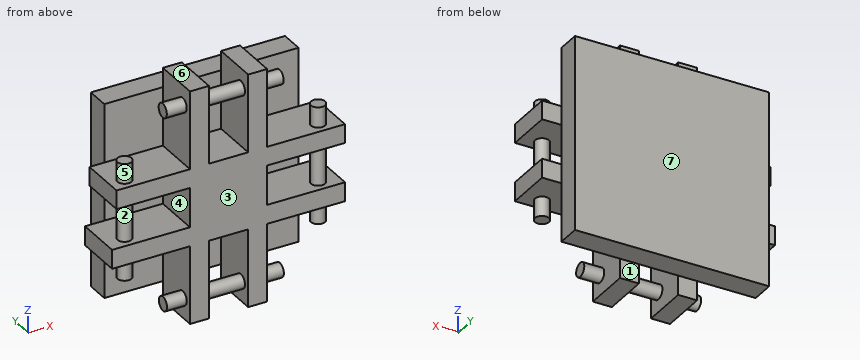
from build123d import *

# Parameters (mm, degrees)
SKETCH1_W                = 79.8
SKETCH1_H                = 79.8
BOSS_EXTRUDE1_DEPTH      = 9.6
SKETCH3_W                = 93.857769302
SKETCH3_H                = 7.7
SKETCH3_W_2              = 31.7
SKETCH3_H_2              = 31.7
SKETCH3_W_3              = 95.7
SKETCH3_H_3              = 7.8
SKETCH3_W_4              = 7.8
SKETCH3_H_4              = 95.7
BOSS_EXTRUDE2_DEPTH      = 19.3
BOSS_EXTRUDE3_DEPTH      = 32
BOSS_EXTRUDE3_DEPTH_BACK = 16
SKETCH4_R                = 2.9
BOSS_EXTRUDE4_DEPTH      = 32
BOSS_EXTRUDE4_DEPTH_BACK = 16
SKETCH5_R                = 2.9
BOSS_EXTRUDE5_DEPTH      = 32
BOSS_EXTRUDE5_DEPTH_BACK = 16
SKETCH6_R                = 2.9
BOSS_EXTRUDE6_DEPTH      = 32
BOSS_EXTRUDE6_DEPTH_BACK = 16
SKETCH7_R                = 2.9


with BuildPart() as part:
    # Sketch1 → Boss-Extrude1 (new body)
    with BuildSketch(Plane(origin=(0, 0, 0), x_dir=(1, 0, 0), z_dir=(0, 1, 0))):
        with Locations((-0.532, -4.965333333)):
            Rectangle(SKETCH1_W, SKETCH1_H)
    extrude(amount=BOSS_EXTRUDE1_DEPTH)

    # Sketch3 → Boss-Extrude2 (add)
    with BuildSketch(Plane.XZ):
        with Locations((0.389115349, 16.965333333)):
            Rectangle(SKETCH3_W, SKETCH3_H)
        with Locations((-0.532, 4.965333333)):
            Rectangle(SKETCH3_W_2, SKETCH3_H_2)
        with Locations((-0.532, -6.984666667)):
            Rectangle(SKETCH3_W_3, SKETCH3_H_3)
        with Locations((-12.482, 4.965333333)):
            Rectangle(SKETCH3_W_4, SKETCH3_H_4)
        with Locations((11.418, 4.965333333)):
            Rectangle(SKETCH3_W_4, SKETCH3_H_4)
    extrude(amount=BOSS_EXTRUDE2_DEPTH)

    # Sketch4 → Boss-Extrude3 (add, two sides: drawn at the far end of the back side and taken through both)
    with BuildSketch(Plane.XY.offset(-3.084666667).offset(-BOSS_EXTRUDE3_DEPTH_BACK)):
        with Locations((-40.282, -14.1)):
            Circle(SKETCH4_R)
    extrude(amount=BOSS_EXTRUDE3_DEPTH + BOSS_EXTRUDE3_DEPTH_BACK)

    # Sketch5 → Boss-Extrude4 (add, two sides: drawn at the far end of the back side and taken through both)
    with BuildSketch(Plane(origin=(-8.582, 0, 0), x_dir=(0, 0, -1), z_dir=(1, 0, 0)).offset(-BOSS_EXTRUDE4_DEPTH_BACK)):
        with Locations((-44.715333333, -14.1)):
            Circle(SKETCH5_R)
    extrude(amount=BOSS_EXTRUDE4_DEPTH + BOSS_EXTRUDE4_DEPTH_BACK)

    # Sketch6 → Boss-Extrude5 (add, two sides: drawn at the far end of the back side and taken through both)
    with BuildSketch(Plane(origin=(0, 0, 13.115333333), x_dir=(-1, 0, 0), z_dir=(0, 0, -1)).offset(-BOSS_EXTRUDE5_DEPTH_BACK)):
        with Locations(Location((-39.218, -14.1, 0), (0, 0, 180))):
            Circle(SKETCH6_R)
    extrude(amount=BOSS_EXTRUDE5_DEPTH + BOSS_EXTRUDE5_DEPTH_BACK)

    # Sketch7 → Boss-Extrude6 (add, two sides: drawn at the far end of the back side and taken through both)
    with BuildSketch(Plane.ZY.offset(-7.518).offset(-BOSS_EXTRUDE6_DEPTH_BACK)):
        with Locations((-34.784666667, -14.1)):
            Circle(SKETCH7_R)
    extrude(amount=BOSS_EXTRUDE6_DEPTH + BOSS_EXTRUDE6_DEPTH_BACK)


solid = part.part
Geometry check sheet. Reference: the model listing, model coordinates, mm. Face numbers are marked on the shaded views. A direction names the side the tool comes from. Give positions to 0.01 mm unless a question says otherwise; leave off trailing zeros. Write each loop counter-clockwise with the first axis right and the second up, starting at its lowest first coordinate (ties: lowest second). Pieces come first, ordered by that corner, then holes.
1) Cross-section at B-B (y = -2.75). Record the boundary of the cut face in (x, z).
Values follow:
outline: (-48.38, -10.88) - (-16.38, -10.88) - (-16.38, -42.88) - (-8.58, -42.88) - (-8.58, -10.88) - (7.52, -10.88) - (7.52, -42.88) - (15.32, -42.88) - (15.32, -10.88) - (47.32, -10.88) - (47.32, -3.08) - (15.32, -3.08) - (15.32, 13.12) - (47.32, 13.12) - (47.32, 20.82) - (15.32, 20.82) - (15.32, 52.82) - (7.52, 52.82) - (7.52, 20.82) - (-8.58, 20.82) - (-8.58, 52.82) - (-16.38, 52.82) - (-16.38, 20.82) - (-46.54, 20.82) - (-46.54, 13.12) - (-16.38, 13.12) - (-16.38, -3.08) - (-48.38, -3.08) - close
2) Thickness scan on line 1 (Z direction, x = -20, y = -8.5); line 2 (X direction, y = -7, z = 25.5); line 3 (Z direction, x = -38.5, y = 4). Record the ranges inside material, lowest first.
Values follow:
line 1: z = -10.88 to -3.08, 13.12 to 20.82
line 2: x = -16.38 to -8.58, 7.52 to 15.32
line 3: z = -34.93 to 44.87
3) Set-up check for the marked faces 1, 2, 3 and 4: record each of +Z, -Z, +X, -X, +Y, -Y from which the full face is reachable in a straight line by a thin tool's end or side.
Values follow:
face 1: -Z, +X, -X, +Y
face 2: none
face 3: +Z, -Z, +X, -X, -Y
face 4: -Y
4) Cross-section at C-C (x = -31). Record the boundary of the cut face in (y, z), plus the area to 3 significant figures.
Values follow:
outline: (-19.3, -10.88) - (0, -10.88) - (0, -34.93) - (9.6, -34.93) - (9.6, 44.87) - (0, 44.87) - (0, 20.82) - (-19.3, 20.82) - (-19.3, 13.12) - (0, 13.12) - (0, -3.08) - (-19.3, -3.08) - close
area: 1,070 mm2
5) Cross-section at A-A (x = -18). Record the boundary of the cut face in (y, z).
Values follow:
outline: (-19.3, -10.88) - (0, -10.88) - (0, -34.93) - (9.6, -34.93) - (9.6, 44.87) - (0, 44.87) - (0, 20.82) - (-19.3, 20.82) - (-19.3, 13.12) - (0, 13.12) - (0, -3.08) - (-19.3, -3.08) - close; circle Ø5.8 at (-14.1, -34.78); circle Ø5.8 at (-14.1, 44.72)
6) Cross-section at D-D (x = 6). Record the boundary of the cut face in (y, z).
Values follow:
outline: (-19.3, -10.88) - (0, -10.88) - (0, -34.93) - (9.6, -34.93) - (9.6, 44.87) - (0, 44.87) - (0, 20.82) - (-19.3, 20.82) - close; circle Ø5.8 at (-14.1, -34.78); circle Ø5.8 at (-14.1, 44.72)
7) Release check for a two-part mould opening along Y. For the marked faces 5, 6 and 7 record: released by +Y, released by -Y, zero draft, split by the parting line, or undercut.
Values follow:
face 5: undercut
face 6: zero draft
face 7: released by +Y
8) Go/stop test with flat-tipped pins: pin 1 Ø4 at (y, z) = (-6, -28) entering from +X; pin 2 Ø13 at (y, z) = (-10, 3.5) entering from +X; pin 3 Ø6.5 at (y, z) = (-13.5, -36) entering from +X. Record where each tip stops, or that it passes through.
Values follow:
pin 1: stops at x = 15.32
pin 2: stops at x = 42.12
pin 3: stops at x = 23.52
